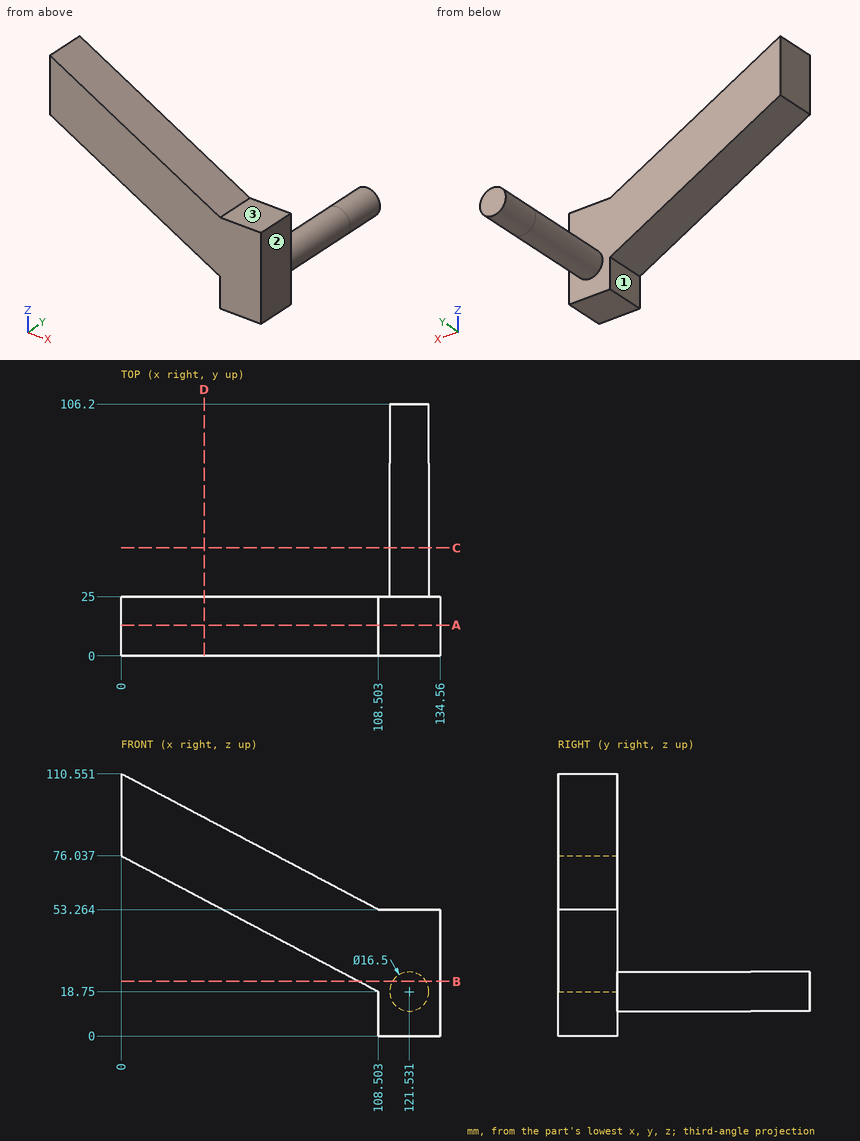
Source: three-view drawing plus pictorial views. Frame: mm from the lowest corner of the part. A direction names the side the tool comes from. Give positions to 0.01 mm unless a question says otherwise; leave off trailing zeros. Write each loop counter-clockwise with the first axis right and the second up, starting at its lowest first coordinate (ties: lowest second). Pieces come first, ordered by that corner, then holes.
(1) Cut plane D-D, the plane x = 35. Return loops of the section in (y, z).
(2) Cut plane C-C, the plane y = 45.5. Return loops of the section in (x, z).
(3) First-contact query: P1, Ø5, axis at x = 18, z = 70.5, coming from the -Y side; P2, Ø5.5, axis at y = 8, z = 9, coming from the -X side; P3, Ø12.5, axis at x = 127.5, y = 9, coming from the +Z side; P4, Ø12, axis at x = 64, z = 40.5, coming from the +Y side. Flat tips, straight axial feed; report the tip coordinate or a pass-through.
(4) Cut plane A-A, the plane y = 13. Return loops of the section in (x, z).
(5) Cut plane B-B, the plane z = 23. Return loops of the section in (x, y).
(6) Ray query, line 1 (Z direction, x = 114.5, y = 8.5); line 2 (Y direction, x = 59.5, z = 76.5); line 3 (X direction, y = 21.5, z = 40.5) (1 decimal). Return the intervals inside material, ascending.
(7) Access query for the marked faces 1, 2 and 3. Directions: +Z, -Z, +X, -X, +Y, -Y. A direction counts if a zero-diameter tool reaches every point of the face in a straight line with its end or side. Return the directions, or none.
Values follow:
1. outline: (0, 57.56) - (25, 57.56) - (25, 92.07) - (0, 92.07) - close
2. outline: circle Ø16.5 at (121.53, 18.75)
3. P1: stops at y = 0
3. P2: stops at x = 108.5
3. P3: stops at z = 53.26
3. P4: stops at y = 25
4. outline: (0, 76.04) - (108.5, 18.75) - (108.5, 0) - (134.56, 0) - (134.56, 53.26) - (108.5, 53.26) - (0, 110.55) - close
5. outline: (100.45, 0) - (134.56, 0) - (134.56, 25) - (128.6, 25) - (128.6, 106.2) - (114.46, 106.2) - (114.46, 25) - (100.45, 25) - close
6. line 1: z = 0 to 53.26
6. line 2: y = 0 to 25
6. line 3: x = 67.3 to 134.6
7. face 1: -Z, -X, +Y, -Y
7. face 2: +Z, -Z, +X, +Y, -Y
7. face 3: +Z, +X, +Y, -Y
